Here's how the part is built. I have some questions about the finished solid (model axes, mm). A direction names the side the tool comes from. Give positions to 0.01 mm unless a question says otherwise; leave off trailing zeros. Loops run counter-clockwise (first coordinate to the right, second up) from the corner with the lowest first, then second, coordinate; pieces in that order, holes last. Notation, with made-up numbers: (-38, 65.5) -> (-9, 65.5) arc R17 cw to (-9, 87.5) -> close; hole circle Ø4 at (-19.75, -18). An arc over 180 degrees is marked (long way). Answer in a Markdown table with one row per item. Add a question column.
Item 1: If I drill on line 1 (Z direction, x = -2.75, y = 1); line 2 (X direction, y = -0.25, z = -30); line 3 (Y direction, x = -0.75, z = 11.5), over which ranges is the centre line in solid material (lowest first)?
Item 2: If we section it at C-C (z = 20): Write out the boundary of the cut face in (x, y).
Item 3: For P1, Ø3, axis at x = -2, z = 0, coming from the -Y side, with a flat end and sliding along its axis, tell me the tip position at first contact or that it passes through.
Item 4: If we section it at A-A (y = 0): Write out the boundary of the cut face in (x, z).
Item 5: Which directions (+Z, -Z, +X, -X, +Y, -Y) give clear straight access to the entire face, cutting with the end or side of a thin tool? Please do faces 1 (the face through (-3.245, 1.022, -37.463)), 2 (the face through (-1.29, 2.024, 40.424)).
```python
from build123d import *

# Parameters (mm, degrees)
SKETCH1_R           = 2.5
BOSS_EXTRUDE1_DEPTH = 40.767
SKETCH2_W           = 0.7
SKETCH2_H           = 0.1
SKETCH4_R           = 3.402225697
BOSS_EXTRUDE2_DEPTH = 6.701877401


with BuildPart() as part:
    # Sketch1 → Boss-Extrude1 (new, symmetric)
    with BuildSketch(Plane.XY):
        with Locations(Location((0, 0, 0), (0, 0, 180))):
            Circle(SKETCH1_R)
    extrude(amount=BOSS_EXTRUDE1_DEPTH, both=True)

    # Sketch2 → Cut-Revolve1 (revolve, cut)
    with BuildSketch(Plane(origin=(0, 0, 0), x_dir=(0, 0, -1), z_dir=(1, 0, 0)), mode=Mode.PRIVATE) as cut_revolve1_sk:
        with Locations((-40.441143952, 2.45)):
            Rectangle(SKETCH2_W, SKETCH2_H)
    revolve(cut_revolve1_sk.sketch.rotate(Axis((0, 0, 40.767), (0, 0, -1)), 270), axis=Axis((0, 0, 40.767), (0, 0, -1)), mode=Mode.SUBTRACT)

    # Sketch4 → Boss-Extrude2 (add)
    with BuildSketch(Plane(origin=(0, 0, -40.767), x_dir=(-1, 0, 0), z_dir=(0, 0, -1))):
        Circle(SKETCH4_R)
    extrude(amount=-BOSS_EXTRUDE2_DEPTH)


solid = part.part
```
Recorded:
| question | item | result |
|---|---|---|
| 1 | line 1 | z = -40.77 to -34.07 |
| 1 | line 2 | x = -2.49 to 2.49 |
| 1 | line 3 | y = -2.38 to 2.38 |
| 2 | outline | circle Ø5 at (0, 0) |
| 3 | P1 | stops at y = -2.45 |
| 4 | outline | (-3.4, -40.77) -> (3.4, -40.77) -> (3.4, -34.07) -> (2.5, -34.07) -> (2.5, 40.09) -> (2.4, 40.09) -> (2.4, 40.77) -> (-2.4, 40.77) -> (-2.4, 40.09) -> (-2.5, 40.09) -> (-2.5, -34.07) -> (-3.4, -34.07) -> close |
| 5 | face 1 | +Z, -Z |
| 5 | face 2 | +Z |
